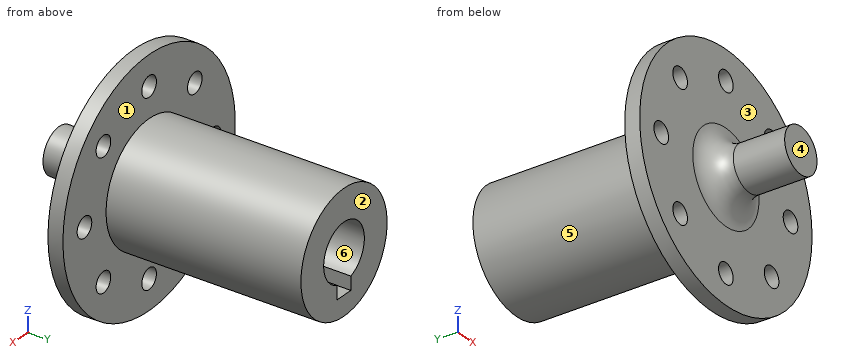
from build123d import *

# Parameters (mm, degrees)
SKETCH1_R                   = 12.7
BOSS_EXTRUDE1_DEPTH         = 41.275
SKETCH3_R                   = 25.4
BOSS_EXTRUDE3_DEPTH         = 3.175
F_8_CLEARANCE_HOLE1_D       = 4.3053
F_20_8MMTOENDOFKEYWAY_DEPTH = 22.0625
SKETCH8_R                   = 4.7625
BOSS_EXTRUDE4_DEPTH         = 15.875
FILLET1_R                   = 5


with BuildPart() as part:
    # Sketch1 → Boss-Extrude1 (new body)
    with BuildSketch(Plane(origin=(0, 0, 0), x_dir=(1, 0, 0), z_dir=(0, 1, 0))):
        Circle(SKETCH1_R)
    extrude(amount=BOSS_EXTRUDE1_DEPTH)

    # Sketch3 → Boss-Extrude3 (add)
    with BuildSketch(Plane.XZ):
        Circle(SKETCH3_R)
    extrude(amount=BOSS_EXTRUDE3_DEPTH)

    # #8 Clearance Hole1 (through all)
    with Locations(Plane(origin=(0, -3.175, 0), x_dir=(-1, 0, 0), z_dir=(0, -1, 0))):
        with Locations((0, 19.05), (-13.470384182, 13.470384182), (-19.05, 0), (-13.470384182, -13.470384182), (0, -19.05), (13.470384182, -13.470384182), (19.05, 0), (13.470384182, 13.470384182)):
            Hole(F_8_CLEARANCE_HOLE1_D / 2)

    # Sketch7 → 20.8mmToEndofKeyway (cut)
    with BuildSketch(Plane(origin=(0, 41.275, 0), x_dir=(1, 0, 0), z_dir=(0, 1, 0))):
        with BuildLine():
            Line((-2, 8.5), (2, 8.5))
            Line((2, 8.5), (2, 5.656854249))
            ThreePointArc((2, 5.656854249), (0, -6), (-2, 5.656854249))
            Line((-2, 5.656854249), (-2, 8.5))
        make_face()
    extrude(amount=-F_20_8MMTOENDOFKEYWAY_DEPTH, mode=Mode.SUBTRACT)

    # Sketch8 → Boss-Extrude4 (add)
    with BuildSketch(Plane.XZ.offset(3.175)):
        Circle(SKETCH8_R)
    extrude(amount=BOSS_EXTRUDE4_DEPTH)

    # Fillet1
    fillet1_edges = [part.edges().sort_by_distance(p)[0] for p in [
        (-4.7625, -3.175, 0),
    ]]
    fillet(fillet1_edges, radius=FILLET1_R)


solid = part.part
Geometry check sheet. Reference: the model listing, model coordinates, mm. Face numbers are marked on the shaded views. A direction names the side the tool comes from. Give positions to 0.01 mm unless a question says otherwise; leave off trailing zeros. Write each loop counter-clockwise with the first axis right and the second up, starting at its lowest first coordinate (ties: lowest second). Pieces come first, ordered by that corner, then holes. Notation, with made-up numbers: M 55.25,23 L 109.25,23 A11 cw 109.25,39 Z; hole C 74,-18 d9. An arc over 180 degrees is marked long. Answer as CSV lines item,"result". Start each with the question number.
Q1. Tool access check on the marked faces 1, 2 and 3. Record the directions out of +Z, -Z, +X, -X, +Y, -Y that give a thin tool (end or side, any length) a straight path to the whole face; none if there is none.
Q2. Section check C-C, the plane x = 19.05. Record the cut outline in (y, z) (3 decimals).
Q3. Release check for a two-part mould opening along Z. For the marked faces 4, 5 and 6 record: pulls with the +Z half, pulls with the -Z half, needs draft (parallel to the pull), parting line crosses it, or undercut.
Q4. Section check A-A, the plane z = 0. Give the number of separate pieces and of enclosed holes in the cut face, then the cut area to 3 significant figures.
Q5. Material ranges on L1, parallel to Y at x = -0.5, z = 0; L2, parallel to Y at x = 13.5, z = 5.5 (3 decimals); L3, parallel to Z at x = 5, y = 24, recorded low to high.
Q6. Go/stop test with flat-tipped pins: pin 1 (3.5 mm diameter, centred on x = 2.5, z = -1, fed in from +Y); pin 2 (5.5 mm diameter, centred on x = 13.47, z = -13.47, fed in from +Y); pin 3 (5 mm diameter, centred on x = -13.47, z = -13.47, fed in from -Y) (3 decimals). Record where each tip stops, or that it passes through.
Geometry says:
1,face 1,"+Y"
1,face 2,"+Z, -Z, +X, -X, +Y"
1,face 3,"-Y"
2,outline,"M -3.175,-16.801 L 0,-16.801 L 0,-2.153 L -3.175,-2.153 Z; M -3.175,2.153 L 0,2.153 L 0,16.801 L -3.175,16.801 Z"
3,face 4,"needs draft"
3,face 5,"parting line crosses it"
3,face 6,"undercut"
4,separate pieces,"3"
4,enclosed holes,"0"
4,area,"1,080 mm^2"
5,L1,"-19.05 to 19.21"
5,L2,"-3.175 to 0"
5,L3,"-11.67 to -3.32, 3.32 to 11.67"
6,pin 1,"y = 19.21"
6,pin 2,"y = 0"
6,pin 3,"y = -3.175"
